Input: part model. Units: mm. Frame: model coordinates. A direction names the side the tool comes from. Coordinates: 2 decimals unless noted, no trailing zeros. Order: outer loops, then holes, each group sorted by start corner. A loop starts at its lowest first (then second) coordinate and runs counter-clockwise, first axis right, second up. Notation, with made-up numbers: (45, 69) - (64, 69) arc R25 cw to (64, 83) - close; hole circle Ø9 at (-27, 0.25). An arc over 180 degrees is marked (long way). Use a Markdown table: item, result. Add a question column.
from build123d import *

# Parameters (mm, degrees)
F0_R     = 2.5
F1_DEPTH = 150


with BuildPart() as f1:
    # F0 (on Right) → F1 (new body)
    with BuildSketch(Plane.YZ):
        with BuildLine():
            ThreePointArc((10.0095693261, 7.9923210088), (9.4265099626, 9.411496018), (8.0095840678, 10))
            Line((8.0095840678, 10), (4.1, 10))
            Line((4.1, 10), (4.1, 9.5))
            Line((4.1, 9.5), (3.6, 9.5))
            Line((3.6, 9.5), (3.6, 8))
            Line((3.6, 8), (5.5, 8))
            Line((5.5, 8), (5.5, 6.9142135624))
            Line((5.5, 6.9142135624), (2.1857864376, 3.6))
            Line((2.1857864376, 3.6), (0, 3.6))
            Line((0, 3.6), (-2.1857864376, 3.6))
            Line((-2.1857864376, 3.6), (-5.5, 6.9142135624))
            Line((-5.5, 6.9142135624), (-5.5, 8))
            Line((-5.5, 8), (-3.6, 8))
            Line((-3.6, 8), (-3.6, 9.5))
            Line((-3.6, 9.5), (-4.1, 9.5))
            Line((-4.1, 9.5), (-4.1, 10))
            Line((-4.1, 10), (-8, 10))
            ThreePointArc((-8, 10), (-9.4142135624, 9.4142135624), (-10, 8))
            Line((-10, 8), (-10, 4.1))
            Line((-10, 4.1), (-9.5, 4.1))
            Line((-9.5, 4.1), (-9.5, 3.6))
            Line((-9.5, 3.6), (-8, 3.6))
            Line((-8, 3.6), (-8, 5.5))
            Line((-8, 5.5), (-6.9142135624, 5.5))
            Line((-6.9142135624, 5.5), (-3.6, 2.1857864376))
            Line((-3.6, 2.1857864376), (-3.6, 0))
            Line((-3.6, 0), (-3.6, -2.1857864376))
            Line((-3.6, -2.1857864376), (-6.9142135624, -5.5))
            Line((-6.9142135624, -5.5), (-8, -5.5))
            Line((-8, -5.5), (-8, -3.6))
            Line((-8, -3.6), (-9.5, -3.6))
            Line((-9.5, -3.6), (-9.5, -4.1))
            Line((-9.5, -4.1), (-10, -4.1))
            Line((-10, -4.1), (-10, -8))
            ThreePointArc((-10, -8), (-9.4142135624, -9.4142135624), (-8, -10))
            Line((-8, -10), (-4.1, -10))
            Line((-4.1, -10), (-4.1, -9.5))
            Line((-4.1, -9.5), (-3.6, -9.5))
            Line((-3.6, -9.5), (-3.6, -8))
            Line((-3.6, -8), (-5.5, -8))
            Line((-5.5, -8), (-5.5, -6.9142135624))
            Line((-5.5, -6.9142135624), (-2.1857864376, -3.6))
            Line((-2.1857864376, -3.6), (0, -3.6))
            Line((0, -3.6), (2.1857864376, -3.6))
            Line((2.1857864376, -3.6), (5.5, -6.9142135624))
            Line((5.5, -6.9142135624), (5.5, -8))
            Line((5.5, -8), (3.6, -8))
            Line((3.6, -8), (3.6, -9.5))
            Line((3.6, -9.5), (4.1, -9.5))
            Line((4.1, -9.5), (4.1, -10))
            Line((4.1, -10), (8, -10))
            ThreePointArc((8, -10), (9.4142135624, -9.4142135624), (10, -8))
            Line((10, -8), (10, -4.1))
            Line((10, -4.1), (9.5, -4.1))
            Line((9.5, -4.1), (9.5, -3.6))
            Line((9.5, -3.6), (8, -3.6))
            Line((8, -3.6), (8, -5.5))
            Line((8, -5.5), (6.9142135624, -5.5))
            Line((6.9142135624, -5.5), (3.6, -2.1857864376))
            Line((3.6, -2.1857864376), (3.6, 0))
            Line((3.6, 0), (3.6, 2.1857864376))
            Line((3.6, 2.1857864376), (6.9142135624, 5.5))
            Line((6.9142135624, 5.5), (8, 5.5))
            Line((8, 5.5), (8, 3.6))
            Line((8, 3.6), (9.5, 3.6))
            Line((9.5, 3.6), (9.5, 4.1))
            Line((9.5, 4.1), (10, 4.1))
            Line((10, 4.1), (10, 5.5))
            Line((10, 5.5), (10.0095693261, 7.9923210088))
        make_face()
        Circle(F0_R, mode=Mode.SUBTRACT)
    extrude(amount=F1_DEPTH)


solid = f1.part
1) Reachability of faces 5 (the flat face through (73.95, 5.234, 3.82)), 6 (the flat face through (74, -10, -6)), 7 (the flat face through (0, -2, 2)), 8 (the flat face through (74, 0, -3.6)), 9 (the flat face through (74, 0, 3.6)) from +Z, -Z, +X, -X, +Y, -Y: full face, straight path, thin tool, end or side. Return the list, or none.
2) Pull-direction query (Y, two-part tool) for faces 1 (the flat face through (74, -3.6, 0)), 2 (the flat face through (74, 10, -6)), 3 (the flat face through (73.95, 5.28, -3.866)), 4 (the flat face through (73.95, -3.866, -5.28)); classes: pulls with the +Y half, pulls with the -Y half, needs draft (parallel to the pull), parting line crosses it, or undercut.
3) Cut plane A-A (z = 0). Return the cut outline in (x, y).
4) Material intervals for L1, parallel to Z at x = 35, y = 0; L2, parallel to Z at x = 98, y = -7.75; L3, parallel to Z at x = 112, y = -4.25, sorted ascending.
5) Contact query for flat-ended pins moving along their axis: P1, Ø0.5, axis at x = 59, z = -7.5, coming from the +Y side; P2, Ø0.8, axis at x = 60.5, y = -9, coming from the -Z side; P3, Ø4, axis at y = 0, z = 0, coming from the +X side; P4, Ø1.3, axis at x = 84.5, y = 0, coming from the -Z side. Output: stop coordinate, or through.
Computed:
| question | item | result |
|---|---|---|
| 1 | face 5 | +X, -X |
| 1 | face 6 | +Z, -Z, +X, -X, -Y |
| 1 | face 7 | +Z, -Z, -X, +Y, -Y |
| 1 | face 8 | -Z, +X, -X |
| 1 | face 9 | +Z, +X, -X |
| 2 | face 1 | pulls with the -Y half |
| 2 | face 2 | pulls with the +Y half |
| 2 | face 3 | undercut |
| 2 | face 4 | undercut |
| 3 | outline | (0, -3.6) - (150, -3.6) - (150, -2.5) - (0, -2.5) - close; (0, 2.5) - (150, 2.5) - (150, 3.6) - (0, 3.6) - close |
| 4 | L1 | z = -3.6 to -2.5, 2.5 to 3.6 |
| 4 | L2 | z = -10 to -5.5, 5.5 to 10 |
| 4 | L3 | z = -10 to -8, -5.66 to -2.84, 2.84 to 5.66, 8 to 10 |
| 5 | P1 | stops at y = 10 |
| 5 | P2 | stops at z = -9.91 |
| 5 | P3 | passes through |
| 5 | P4 | stops at z = -3.6 |
